Geometry: final body of the model. Coordinates: model frame, mm. Give positions to 0.01 mm unless a question says otherwise; leave off trailing zeros. Write each loop counter-clockwise with the first axis right and the second up, starting at its lowest first coordinate (ties: lowest second). Pieces come first, ordered by that corner, then holes. Notation, with made-up numbers: (-7.75, 60.5) -> (30.25, 60.5) arc R29 cw to (30.25, 99.5) -> close; hole circle Ø8 at (61, -19). An arc over 180 degrees is marked (long way). Use CSV: the item, a comma, the result in double quotes. Start each with the question number.
1) Section A-A (x = -23.5). Output: boundary loops of the cut face in (y, z).
2) Contact query for a flat-ended pin moving along its axis: P1, Ø2, axis at x = 4.5, z = 6, coming from the -Y side (3 decimals). Output: stop coordinate, or through.
3) Section D-D (y = 1.45). Output: boundary loops of the cut face in (x, z), plus the area to 3 significant figures.
4) Section C-C (x = -44.5). Output: boundary loops of the cut face in (y, z), plus the area to 3 significant figures.
5) Section B-B (z = 6). Output: boundary loops of the cut face in (x, y).
6) Material intervals for line 1 (Z direction, x = -44.5, y = 2.25); line 2 (X direction, y = 1.3, z = 6); line 3 (X direction, y = 1, z = -51), sorted ascending. Write a range as [from, to].
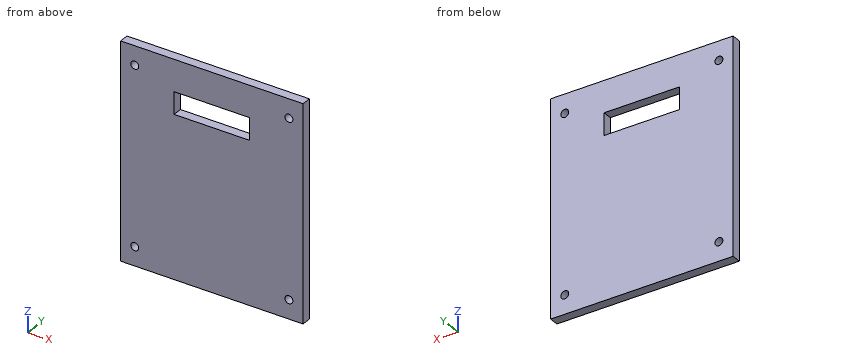
Autodesk Inventor part; units mm, degrees
ref_plane "YZ Plane" through (0, 0, 0) normal (1, 0, 0) x (0, 1, 0)
ref_plane "XZ Plane" through (0, 0, 0) normal (0, 1, 0) x (-1, 0, 0)
ref_plane "XY Plane" through (0, 0, 0) normal (0, 0, 1) x (1, 0, 0)
sketch "Sketch2" plane through (0, 0, 0) normal (0, 1, 0) x (-1, 0, 0)
  line L0 (8, 0) -> (8, -5)
  line L1 (32, 0) -> (32, -5)
  line L2 (32, -5) -> (8, -5)
  line L3 (8, -5) -> (8, 0)
  line L4 (32, 0) -> (32, -5)
  line L5 (-9, 0) -> (-9, 9)
  line L6 (-9, 9) -> (0, 9)
  line L7 (49, -44) -> (49, -53)
  line L8 (49, -53) -> (40, -53)
  line L9 (-9, 9) -> (49, 9)
  line L10 (49, 9) -> (49, -53)
  line L11 (49, -53) -> (-9, -53)
  line L12 (-9, -53) -> (-9, 9)
  line L13 (8, 0) -> (8, 2)
  line L14 (8, 2) -> (32, 2)
  line L15 (32, 2) -> (32, 0)
  line L16 (32, 2) -> (8, 2)
  line L17 (8, 2) -> (8, -5)
  line L18 (8, -5) -> (32, -5)
  line L19 (32, -5) -> (32, 2)
  point P0 (0, 0)
extrude "Extrusion1" add sketch "Sketch2" along normal blind 3
sketch "Sketch3" plane through (-49, 0, 9) normal (0, 0, 1) x (1, 0, 0)
  line L0 (0, 0) -> (0, 3)
  line L1 (58, 0) -> (58, 3)
  line L2 (0, 3) -> (58, 3)
  line L3 (58, 3) -> (58, 0)
  line L4 (58, 0) -> (0, 0)
  line L5 (0, 0) -> (0, 3)
  point P0 (49, 0)
extrude "Extrusion2" add sketch "Sketch3" along normal blind 3
sketch "Sketch4" plane through (9, 0, -53) normal (0, 0, -1) x (-1, 0, 0)
  line L0 (58, 3) -> (58, 0)
  line L1 (58, 0) -> (0, 0)
  line L2 (58, 3) -> (0, 3)
  line L3 (0, 3) -> (0, 0)
  line L4 (0, 0) -> (58, 0)
  line L5 (58, 0) -> (58, 3)
  point P0 (9, 0)
extrude "Extrusion3" add sketch "Sketch4" along normal blind 3
sketch "Sketch5" plane through (0, 3, 0) normal (0, 1, 0) x (1, 0, 0)
  line L0 (9, -12) -> (0, -12)
  line L1 (0, -12) -> (0, 0)
  line L2 (0, 0) -> (9, 0)
  line L3 (9, 0) -> (9, -12)
  line L4 (-49, -12) -> (-49, 56)
  line L5 (-49, 56) -> (-40, 56)
  line L6 (-40, 56) -> (-40, 44)
  line L7 (-40, 44) -> (-49, 44)
  line L8 (-49, 44) -> (-49, 56)
  line L9 (9, 56) -> (0, 56)
  line L10 (0, 56) -> (0, 44)
  line L11 (0, 44) -> (9, 44)
  line L12 (9, 44) -> (9, 56)
  circle A0 centre (-44.5, 50) radius 1.25
  circle A1 centre (4.5, 50) radius 1.25
  circle A2 centre (4.5, -6) radius 1.25
  line L13 (-49, -12) -> (-40, -12)
  line L14 (-40, -12) -> (-40, 0)
  line L15 (-40, 0) -> (-49, 0)
  line L16 (-49, 0) -> (-49, -12)
  circle A3 centre (-44.5, -6) radius 1.25
  dimension "d16" = 9
  dimension "d17" = 12
  dimension "d18" = 9
  dimension "d19" = 12
  dimension "d21" = 2.5
  dimension "d22" = 2.5
  dimension "d23" = 2.5
  dimension "d24" = 2.5
extrude "Extrusion4" cut sketch "Sketch5" against normal blind 5 contours A0 | A1 | A2 | A3
properties part number "Podkladka"
Answers follow:
1,outline,"(0, -56) -> (3, -56) -> (3, -5) -> (0, -5) -> close; (0, 2) -> (3, 2) -> (3, 12) -> (0, 12) -> close"
2,P1,"passes through"
3,outline,"(-49, -56) -> (9, -56) -> (9, 12) -> (-49, 12) -> close; hole circle Ø2.5 at (-44.5, -50); hole circle Ø2.5 at (-44.5, 6); hole (-32, -5) -> (-8, -5) -> (-8, 2) -> (-32, 2) -> close; hole circle Ø2.5 at (4.5, -50); hole circle Ø2.5 at (4.5, 6)"
3,area,"3,760 mm^2"
4,outline,"(0, -56) -> (3, -56) -> (3, -51.25) -> (0, -51.25) -> close; (0, -48.75) -> (3, -48.75) -> (3, 4.75) -> (0, 4.75) -> close; (0, 7.25) -> (3, 7.25) -> (3, 12) -> (0, 12) -> close"
4,area,"189 mm^2"
5,outline,"(-49, 0) -> (-45.75, 0) -> (-45.75, 3) -> (-49, 3) -> close; (-43.25, 0) -> (3.25, 0) -> (3.25, 3) -> (-43.25, 3) -> close; (5.75, 0) -> (9, 0) -> (9, 3) -> (5.75, 3) -> close"
6,line 1,"z = [-56, -51.25], [-48.75, 4.75], [7.25, 12]"
6,line 2,"x = [-49, -45.75], [-43.25, 3.25], [5.75, 9]"
6,line 3,"x = [-49, -45.25], [-43.75, 3.75], [5.25, 9]"
